from build123d import *

# Parameters (mm, degrees)
SKETCH1_W           = 1670.558
SKETCH1_H           = 800.1
BOSS_EXTRUDE1_DEPTH = 457.2
CUT_EXTRUDE1_DEPTH  = 457.2


with BuildPart() as part:
    # Sketch1 → Boss-Extrude1 (new body)
    with BuildSketch(Plane.XY):
        with Locations((-20.24385353, 108.686840885)):
            Rectangle(SKETCH1_W, SKETCH1_H)
    extrude(amount=BOSS_EXTRUDE1_DEPTH)

    # Sketch2 → Cut-Extrude1 (cut)
    with BuildSketch(Plane.XY.offset(457.2)):
        Polygon((506.93314647, 508.736840885), (506.93314647, 464.286840885), (431.24114647, 464.286840885), (431.24114647, 419.836840885), (355.54914647, 419.836840885), (355.54914647, 375.386840885), (279.85714647, 375.386840885), (279.85714647, 330.936840885), (204.16514647, 330.936840885), (204.16514647, 286.486840885), (128.47314647, 286.486840885), (128.47314647, 242.036840885), (52.78114647, 242.036840885), (52.78114647, 197.586840885), (-22.91085353, 197.586840885), (-22.91085353, 153.136840885), (-98.60285353, 153.136840885), (-98.60285353, 108.686840885), (-174.29485353, 108.686840885), (-174.29485353, 64.236840885), (-249.98685353, 64.236840885), (-249.98685353, 19.786840885), (-325.67885353, 19.786840885), (-325.67885353, -24.663159115), (-401.37085353, -24.663159115), (-401.37085353, -69.113159115), (-477.06285353, -69.113159115), (-477.06285353, -113.563159115), (-552.75485353, -113.563159115), (-552.75485353, -158.013159115), (-628.44685353, -158.013159115), (-628.44685353, -202.463159115), (-704.13885353, -202.463159115), (-704.13885353, -246.913159115), (-779.83085353, -246.913159115), (-779.83085353, -291.363159115), (-855.52285353, -291.363159115), (-855.52285353, 508.736840885), align=None)
    extrude(amount=-CUT_EXTRUDE1_DEPTH, mode=Mode.SUBTRACT)


solid = part.part
Work out the finished part from the listing and answer in its coordinate system (mm). A direction names the side the tool comes from. Give positions to 0.01 mm unless a question says otherwise; leave off trailing zeros. Write each loop counter-clockwise with the first axis right and the second up, starting at its lowest first coordinate (ties: lowest second). Pieces come first, ordered by that corner, then holes. Notation, with made-up numbers: M -20.75,-1 L 35.25,-1 A12 cw 35.25,22 Z; hole C 43.5,5 d5. An arc over 180 degrees is marked long. Answer as CSV lines item,"result".
Q1. A tool of negligible diameter and unlimited length cuts with its end or side. For faces 1 (the flat face through (6, -291.363, 225)), 2 (the flat face through (128.473, 265, 232)), from which of +Z, -Z, +X, -X, +Y, -Y can it reach the whole face along a straight path? Write none if from no direction.
A:
face 1,"+Z, -Z, +X, -X, -Y"
face 2,"+Z, -Z, -X, +Y"
Q2. A cutting plane is placed at A-A on x = -290. Write down the section's boundary in (y, z).
A:
outline,"M -291.36,0 L 19.79,0 L 19.79,457.2 L -291.36,457.2 Z"
Q3. Given P1, Ø12, axis at x = 271, z = 154.5, coming from the +Y side; P2, Ø22, axis at y = 49, z = 309, coming from the -X side; P3, Ø2, axis at x = 327, z = 159.5, coming from the +Y side, each flat-ended and moving along its own axis, determine where each tip first touches the part or whether it passes through.
A:
P1,"stops at y = 330.94"
P2,"stops at x = -249.99"
P3,"stops at y = 375.39"
Q4. Find the intervals of material crossed by probe 1 along X at (y, z) = (139, 267); probe 2 along X at (y, z) = (72, 121); probe 3 along Y at (x, z) = (-151.5, 42), in increasing order. Write a range as [from, to].
A:
probe 1,"x = [-98.6, 815.04]"
probe 2,"x = [-174.29, 815.04]"
probe 3,"y = [-291.36, 108.69]"
Q5. A cutting plane is placed at B-B on y = 86. Write down the section's boundary in (x, z), plus the area to 3 significant figures.
A:
outline,"M -174.29,0 L 815.04,0 L 815.04,457.2 L -174.29,457.2 Z"
area,"452,000 mm²"
